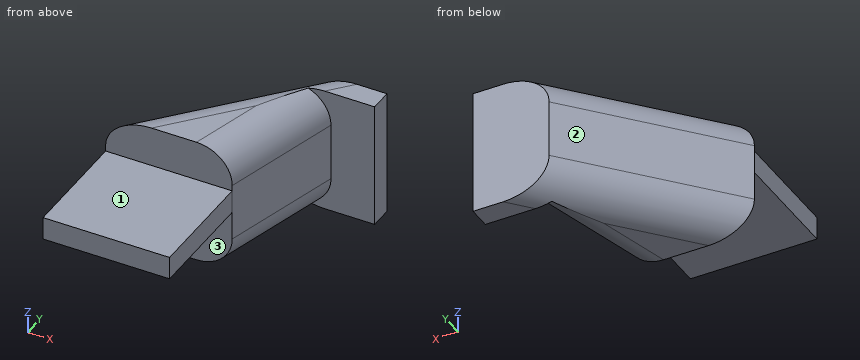
from build123d import *

# Parameters (mm, degrees)
F0_W         = 22
F0_H         = 20
F1_DEPTH     = 4
F2_DEPTH     = 11
F3_DEPTH     = 11
F4_T1_DEPTH  = 63.4073519566
F4_T6_DEPTH  = 51.9365723987
F4_T11_DEPTH = 51.9365723987


# Not quite as in the source:
# - a fillet or chamfer that OpenCascade refuses, or shapes differently, is made with other operations: its cross-section is extruded or revolved along the edge and cut away or added


with BuildPart() as f1:
    # F0 (on Top) → F1 (new body)
    with BuildSketch(Plane.XY):
        with Locations((-11, 10)):
            Rectangle(F0_W, F0_H)
    extrude(amount=F1_DEPTH)

    # F0 (on Top) → F2 (join)
    with BuildSketch(Plane.XY):
        Polygon((-22, 20), (0, 20), (5.6250016205, 41.2031263113), (13.2187530398, 41.2031263113), (13.2187530398, 45.1406277716), (0, 45.1406277716), align=None)
    extrude(amount=F2_DEPTH)

    # F0 (on Top) → F3 (join)
    with BuildSketch(Plane.XY):
        Polygon((-22, 20), (0, 20), (5.6250016205, 41.2031263113), (13.2187530398, 41.2031263113), (13.2187530398, 45.1406277716), (0, 45.1406277716), align=None)
    extrude(amount=-F3_DEPTH)

    # F4: fillet of radius 6 on 4 edges, made by hand

    # F4_s2 → F4_t1 (cut)
    with BuildSketch(Plane(origin=(32.2489050023, 36.8526234865, 0), x_dir=(0, 0, 1), z_dir=(-0.6585376784, -0.7525477567, 0))):
        with BuildLine():
            ThreePointArc((-5, 29.7268042156), (-9.2426406871, 27.9694449027), (-11, 23.7268042156))
            Line((-11, 23.7268042156), (-11, 29.7268042156))
            Line((-11, 29.7268042156), (-5, 29.7268042156))
        make_face()
        with BuildLine():
            ThreePointArc((5, 29.7268042156), (9.2426406871, 27.9694449027), (11, 23.7268042156))
            Line((11, 23.7268042156), (11, 29.7268042156))
            Line((11, 29.7268042156), (5, 29.7268042156))
        make_face()
    extrude(amount=F4_T1_DEPTH, mode=Mode.SUBTRACT)


with BuildPart() as f4_tool4:
    # F4_s5 → F4_t6 (new body)
    with BuildSketch(Plane(origin=(1.1106377761, 4.1864864479, 0), x_dir=(0, 0, 1), z_dir=(0.2564211727, 0.9665651464, 0))):
        with BuildLine():
            ThreePointArc((-11, -11.1284234549), (-9.2426406871, -6.8857827678), (-5, -5.1284234549))
            Line((-5, -5.1284234549), (-11, -5.1284234549))
            Line((-11, -5.1284234549), (-11, -11.1284234549))
        make_face()
    extrude(amount=F4_T6_DEPTH)

    split(bisect_by=Plane.XZ.offset(-41.2031263113), keep=Keep.TOP)


with BuildPart() as f1_1:
    add(f1.part)

    # F4_t3: cut F4_tool4
    add(f4_tool4.part, mode=Mode.SUBTRACT)


with BuildPart() as f4_tool9:
    # F4_s10 → F4_t11 (new body)
    with BuildSketch(Plane(origin=(1.1106377761, 4.1864864479, 0), x_dir=(0, 0, 1), z_dir=(0.2564211727, 0.9665651464, 0))):
        with BuildLine():
            ThreePointArc((11, -11.1284234549), (9.2426406871, -6.8857827678), (5, -5.1284234549))
            Line((5, -5.1284234549), (11, -5.1284234549))
            Line((11, -5.1284234549), (11, -11.1284234549))
        make_face()
    extrude(amount=F4_T11_DEPTH)

    split(bisect_by=Plane.XZ.offset(-41.2031263113), keep=Keep.TOP)


with BuildPart() as f1_2:
    add(f1_1.part)

    # F4_t8: cut F4_tool9
    add(f4_tool9.part, mode=Mode.SUBTRACT)


solid = f1_2.part
Design review of the part built by this model. Coordinates are the model's own, in mm. Face numbers are marked on the shaded views. A direction names the side the tool comes from. Round coordinates to 2 decimals unless told otherwise and drop trailing zeros. Write each loop counter-clockwise with the first axis right and the second up, starting at its lowest first coordinate (ties: lowest second). Pieces come first, ordered by that corner, then holes. Notation, with made-up numbers: (88.5, 47) - (129.5, 47) arc R24 ccw to (129.5, 66) - close; hole circle Ø4 at (-0.75, -39.5). An arc over 180 degrees is marked (long way). Return JSON: item names as keys, results as strings. Group by question number.
Item 1: We need section B-B on x = 11.5. Write out the cut boundary in (y, z).
Item 2: For probe 1 along X at (y, z) = (16, 0.75); probe 2 along Y at (x, z) = (6.5, 1.75); probe 3 along Z at (x, y) = (-4.5, 10), list the stretches that pass through material, from the lowest coordinate up. Write a range as [from, to].
Item 3: We need section C-C on y = 15. Write out the cut boundary in (x, z).
Item 4: Machinability: for the marked faces 1, 2 and 3, which of the approach directions +Z, -Z, +X, -X, +Y, -Y give a long, thin tool a straight path to every point of the face, cutting with its end or side? Answer none if there is none.
Item 5: We need section D-D on z = -1.25. Write out the cut boundary in (x, y) (3 decimals).
Item 6: Insertion check: P1, Ø10, axis at x = -2.5, y = 9, coming from the +Z side; P2, Ø5.5, axis at x = -13, z = -4.5, coming from the -Y side; P3, Ø4, axis at y = 30.5, z = -8.5, coming from the +X side. Each pin has a flat end and moves straight along its axis. Give the tip position at first contact, or say it passes through.
Item 7: We need section A-A on z = 1. Write out the cut boundary in (x, y) (3 decimals), and give its area (3 significant figures).
Model answer:
{
 "1": {"outline": "(41.2, -11) - (45.14, -11) - (45.14, 11) - (41.2, 11) - close"},
 "2": {"probe 1": "x = [-22, 0]", "probe 2": "y = [41.2, 45.14]", "probe 3": "z = [0, 4]"},
 "3": {"outline": "(-22, 0) - (0, 0) - (0, 4) - (-22, 4) - close"},
 "4": {"face 1": "+Z, +X, -X, -Y", "face 2": "+Z, -Z, -X, +Y", "face 3": "-Z, +X, -X, -Y"},
 "5": {"outline": "(-22, 20) - (0, 20) - (5.625, 41.203) - (13.219, 41.203) - (13.219, 45.141) - (0, 45.141) - close"},
 "6": {"P1": "stops at z = 4", "P2": "stops at y = 20", "P3": "stops at x = 2.78"},
 "7": {"outline": "(-22, 0) - (0, 0) - (0, 20) - (5.625, 41.203) - (13.219, 41.203) - (13.219, 45.141) - (0, 45.141) - (-22, 20) - close", "area": "828 mm²"}
}
